```python
from build123d import *
from build123d import SkipClean  # not in build123d's __all__

# Parameters (mm, degrees)
F1_DEPTH  = 108
F3_DEPTH  = 105
F4_W      = 6.2
F4_H      = 3.3
F5_DEPTH  = 4
F4_R      = 3.3
F6_DEPTH  = 2.5
F8_DEPTH  = 1.5
F4_R_2    = 1.5
F9_DEPTH  = 4
F10_W     = 13
F10_H     = 6
F10_W_2   = 6.2
F10_H_2   = 3.3
F11_DEPTH = 3
F10_W_3   = 2
F12_DEPTH = 3
F14_DEPTH = 10
F15_DEPTH = 10


# Not quite as in the source:
# - a feature names something its author has since deleted; it is built from what else it names


with BuildPart() as f1:
    # F0 (on Top) → F1 (new body)
    with BuildSketch(Plane.XY):
        with BuildLine():
            ThreePointArc((6.7082039325, -22), (18.4836237038, -13.6877921805), (23, 0))
            ThreePointArc((23, 0), (20.7160551802, 9.9922498854), (14.3178210633, 18))
            Line((14.3178210633, 18), (-14.3178210633, 18))
            ThreePointArc((-14.3178210633, 18), (-22.5947655837, -4.2984378813), (-6.7082039325, -22))
            Line((-6.7082039325, -22), (6.7082039325, -22))
        make_face()
    extrude(amount=F1_DEPTH)

    # F2 (on face) → F3 (cut)
    with BuildSketch(Plane.XY.offset(108)):
        with BuildLine():
            Line((-6.0827625303, -18), (6.0827625303, -18))
            ThreePointArc((6.0827625303, -18), (18.5894391984, -3.9284539311), (12.8452325787, 14))
            Line((12.8452325787, 14), (-12.8452325787, 14))
            ThreePointArc((-12.8452325787, 14), (-18.5894391984, -3.9284539311), (-6.0827625303, -18))
        make_face()
    extrude(amount=-F3_DEPTH, mode=Mode.SUBTRACT)

    # F4 (on face) → F5 (cut)
    with BuildSketch(Plane(origin=(0, 18, 0), x_dir=(-1, 0, 0), z_dir=(0, 1, 0))):
        with Locations((0, 98.25)):
            Rectangle(F4_W, F4_H)
    extrude(amount=-F5_DEPTH, mode=Mode.SUBTRACT)

    # F4 (on face) → F6 (cut)
    with BuildSketch(Plane(origin=(0, 18, 0), x_dir=(-1, 0, 0), z_dir=(0, 1, 0))):
        with Locations((0, 89.3424802274)):
            Circle(F4_R)
    extrude(amount=-F6_DEPTH, mode=Mode.SUBTRACT)

    # F7 (on face) → F8 (cut)
    with BuildSketch(Plane(origin=(0, 15.5, 0), x_dir=(-1, 0, 0), z_dir=(0, 1, 0))):
        with BuildLine():
            ThreePointArc((3.3, 89.3424802274), (3.2424742607, 89.9559626385), (3.0719026249, 90.5480565471))
            Line((3.0719026249, 90.5480565471), (-3.0719026249, 90.5480565471))
            ThreePointArc((-3.0719026249, 90.5480565471), (-3.3, 89.3424802274), (-3.0719026249, 88.1369039076))
            Line((-3.0719026249, 88.1369039076), (3.0719026249, 88.1369039076))
            ThreePointArc((3.0719026249, 88.1369039076), (3.2424742607, 88.7289978162), (3.3, 89.3424802274))
        make_face()
    extrude(amount=-F8_DEPTH, mode=Mode.SUBTRACT)

    # F4 (on face) → F9 (cut)
    with BuildSketch(Plane(origin=(0, 18, 0), x_dir=(-1, 0, 0), z_dir=(0, 1, 0))):
        with Locations((0, 105)):
            Circle(F4_R_2)
    extrude(amount=-F9_DEPTH, mode=Mode.SUBTRACT)

    # F10 (on face) → F11 (cut)
    with BuildSketch(Plane.XZ.offset(-14)):
        with Locations((0, 98.25)):
            Rectangle(F10_W, F10_H)
        with Locations((0, 98.25)):
            Rectangle(F10_W_2, F10_H_2, mode=Mode.SUBTRACT)
    extrude(amount=-F11_DEPTH, mode=Mode.SUBTRACT)

    # F10 (on face) → F12 (join)
    with BuildSketch(Plane.XZ.offset(-14)):
        with Locations((-7.5, 98.25)):
            Rectangle(F10_W_3, F10_H)
        with Locations((7.5, 98.25)):
            Rectangle(F10_W_3, F10_H)
    extrude(amount=F12_DEPTH)

    # F13 (on face) → F14 (cut)
    with BuildSketch(Plane.XY.offset(108)):
        with BuildLine():
            ThreePointArc((21.2504766076, 0), (20.3841146719, 1.1896729952), (18.9859616706, 0.7302461521))
            ThreePointArc((18.9859616706, 0.7302461521), (18.9964900935, 0.3651905384), (19, 0))
            ThreePointArc((19, 0), (18.9964900935, -0.3651905384), (18.9859616706, -0.7302461521))
            ThreePointArc((18.9859616706, -0.7302461521), (20.3841146719, -1.1896729952), (21.2504766076, 0))
        make_face()
        with BuildLine():
            ThreePointArc((-18.9859616706, -0.7302461521), (-19, 0), (-18.9859616706, 0.7302461521))
            ThreePointArc((-18.9859616706, 0.7302461521), (-21.2504766076, 0), (-18.9859616706, -0.7302461521))
        make_face()
    extrude(amount=-F14_DEPTH, mode=Mode.SUBTRACT)

    # F13 (on face) → F15 (join)
    with BuildSketch(Plane.XY.offset(108)):
        with BuildLine():
            ThreePointArc((18.9859616706, 0.7302461521), (18.9079014817, 1.8684917869), (18.7616630393, 3))
            Line((18.7616630393, 3), (17.0004766076, 3))
            Line((17.0004766076, 3), (17.0004766076, -3))
            Line((17.0004766076, -3), (18.7616630393, -3))
            ThreePointArc((18.7616630393, -3), (18.9079014817, -1.8684917869), (18.9859616706, -0.7302461521))
            ThreePointArc((18.9859616706, -0.7302461521), (18.7504766076, 0), (18.9859616706, 0.7302461521))
        make_face()
        with BuildLine():
            Line((-17.0004766076, 3), (-18.7616630393, 3))
            ThreePointArc((-18.7616630393, 3), (-18.9079014817, 1.8684917869), (-18.9859616706, 0.7302461521))
            ThreePointArc((-18.9859616706, 0.7302461521), (-18.8108036123, 0.3836380643), (-18.7504766076, 0))
            ThreePointArc((-18.7504766076, 0), (-18.8108036123, -0.3836380643), (-18.9859616706, -0.7302461521))
            ThreePointArc((-18.9859616706, -0.7302461521), (-18.9079014817, -1.8684917869), (-18.7616630393, -3))
            Line((-18.7616630393, -3), (-17.0004766076, -3))
            Line((-17.0004766076, -3), (-17.0004766076, 3))
        make_face()
    with SkipClean():  # cleaning this boolean's faces spoils the solid; the shape is the same uncleaned
        extrude(amount=-F15_DEPTH)


solid = f1.part
```
Build history of the part. All positions in model axes, mm. A direction names the side the tool comes from. Round coordinates to 2 decimals unless told otherwise and drop trailing zeros. Loops run counter-clockwise (first coordinate to the right, second up) from the corner with the lowest first, then second, coordinate; pieces in that order, holes last.
Item 1: Two-plate mould, pull along X, no slides. Class faces 4 (the face through (-17, 0, 103)), 5 (the face through (0, -22, 53)), 6 (the face through (-22.66, -3.95, 53.24)): released by +X, released by -X, zero draft, split by the parting line, or undercut.
Item 2: Saw through at A-A (x = 0). List the corners of the cut face in (y, z), then the cut area to 3 significant figures.
Item 3: Pin check, flat tips, straight feed: P1, Ø0.6, axis at x = -8, y = 12, coming from the +Z side; P2, Ø0.5, axis at y = 17.5, z = 97.5, coming from the +X side; P3, Ø12, axis at y = 12, z = 19, coming from the +X side. Stop position of each tip, or through.
Item 4: Drill centre lines: line 1 along Z through (x, y) = (0, 16.4); line 2 along Z through (x, y) = (0, 15); line 3 along X through (y, z) = (0.5, 25.5). Where is each one in solid material? Low to high.
Item 5: Saw through at B-B (z = 105). List the corners of the cut face in (x, y).
Item 6: Saw through at D-D (y = -13.5). List the corners of the cut face in (x, z).
Item 7: Saw through at C-C (z = 57.5). List the corners of the cut face in (x, y), then the cut area to 3 significant figures.
Item 8: Which spindle directions (+Z, -Z, +X, -X, +Y, -Y) get a long thin tool onto all of the face, cutting with end or side? Do faces 1 (the face through (-8, 11, 98)), 2 (the face through (0, -2, 0)), 3 (the face through (-18, 0, 98)). Say none if no direction does.
Worked answers:
1. face 4: undercut
1. face 5: zero draft
1. face 6: released by -X
2. outline: (-22, 0) - (18, 0) - (18, 86.04) - (15.5, 86.04) - (15.5, 88.14) - (14, 88.14) - (14, 3) - (-18, 3) - (-18, 108) - (-22, 108) - close; (14, 90.55) - (15.5, 90.55) - (15.5, 92.64) - (18, 92.64) - (18, 96.6) - (17, 96.6) - (17, 95.25) - (14, 95.25) - close; (14, 101.25) - (17, 101.25) - (17, 99.9) - (18, 99.9) - (18, 103.5) - (14, 103.5) - close; (14, 106.5) - (18, 106.5) - (18, 108) - (14, 108) - close
2. area: 907 mm2
3. P1: stops at z = 101.25
3. P2: stops at x = 15.21
3. P3: stops at x = 22.2
4. line 1: z = 0 to 86.04, 92.64 to 95.25, 101.25 to 103.5, 106.5 to 108
4. line 2: z = 0 to 88.14, 90.55 to 95.25, 101.25 to 103.5, 106.5 to 108
4. line 3: x = -22.99 to -18.99, 18.99 to 22.99
5. outline: (-18.76, -3) - (-17, -3) - (-17, 3) - (-18.76, 3) arc R19 cw to (-12.85, 14) - (-1.5, 14) - (-1.5, 18) - (-14.32, 18) arc R23 ccw to (-6.71, -22) - (6.71, -22) arc R23 ccw to (14.32, 18) - (1.5, 18) - (1.5, 14) - (12.85, 14) arc R19 cw to (18.76, 3) - (17, 3) - (17, -3) - (18.76, -3) arc R19 cw to (6.08, -18) - (-6.08, -18) arc R19 cw to start; hole circle Ø2.5 at (-20, 0); hole circle Ø2.5 at (20, 0)
6. outline: (-18.62, 0) - (18.62, 0) - (18.62, 108) - (13.37, 108) - (13.37, 3) - (-13.37, 3) - (-13.37, 108) - (-18.62, 108) - close
7. outline: (-14.32, 18) arc R23 ccw to (-6.71, -22) - (6.71, -22) arc R23 ccw to (14.32, 18) - close; hole (-12.85, 14) arc R19 ccw to (-6.08, -18) - (6.08, -18) arc R19 ccw to (12.85, 14) - close
7. area: 517 mm2
8. face 1: +Z
8. face 2: -Z, +X, -X, +Y, -Y
8. face 3: none
